Work out the finished part from the listing and answer in its coordinate system (mm). Round coordinates to 2 decimals unless told otherwise and drop trailing zeros. Loops run counter-clockwise (first coordinate to the right, second up) from the corner with the lowest first, then second, coordinate; pieces in that order, holes last. Notation, with made-up numbers: (-5.75, 83) -> (41.25, 83) arc R11 ccw to (41.25, 87) -> close; hole circle Ø7 at (57.5, 10). An arc over 180 degrees is marked (long way). Write item = value, one per line. Start each with the question number.
```python
from build123d import *

# Parameters (mm, degrees)
EXTRUDE_1_DEPTH       = 240
SHEET_START           = -240
SHEET_METAL_1_DEPTH   = 480
SHEET_METAL_1_2_DEPTH = 480
CUT_EXTRUDE_1_REACH   = 247.072
SKETCH_7_R            = 2.5


# Read off the part's stored shape, not the designer's step: Преобразовать-Твердое тело1
with BuildPart() as part:
    # Sketch 1 → Вытянуть-Тонкостенный1 (new, symmetric)
    with BuildSketch(Plane(origin=(0, 0, 0), x_dir=(0, 0, -1), z_dir=(1, 0, 0))):
        Polygon((-19.047619048, 27.896825397), (-19.047619048, 37.896825397), (12.952380952, 37.896825397), (12.952380952, -12.103174603), (2.952380952, -12.103174603), (2.952380952, -10.103174603), (10.952380952, -10.103174603), (10.952380952, 35.896825397), (-17.047619048, 35.896825397), (-17.047619048, 27.896825397), align=None)
    extrude(amount=EXTRUDE_1_DEPTH, both=True)

    # Sheet Metal 1 outline → Sheet Metal 1 (cut)
    with BuildSketch(Plane.YZ.offset(SHEET_START)):
        with BuildLine():
            Line((-12.103174603, -12.952380952), (-8.103174603, -12.952380952))
            ThreePointArc((-8.103174603, -12.952380952), (-10.931601728, -11.780808077), (-12.103174603, -8.952380952))
            Line((-12.103174603, -8.952380952), (-12.103174603, -12.952380952))
        make_face()
        with BuildLine():
            ThreePointArc((33.896825397, 19.047619048), (36.725252521, 17.876046172), (37.896825397, 15.047619048))
            Line((37.896825397, 15.047619048), (37.896825397, 19.047619048))
            Line((37.896825397, 19.047619048), (33.896825397, 19.047619048))
        make_face()
        with BuildLine():
            ThreePointArc((37.896825397, -8.952380952), (36.725252522, -11.780808077), (33.896825397, -12.952380952))
            Line((33.896825397, -12.952380952), (37.896825397, -12.952380952))
            Line((37.896825397, -12.952380952), (37.896825397, -8.952380952))
        make_face()
    extrude(amount=SHEET_METAL_1_DEPTH, mode=Mode.SUBTRACT)

    # Sheet Metal 1 2 outline → Sheet Metal 1 2 (add)
    with BuildSketch(Plane.YZ.offset(SHEET_START)):
        with BuildLine():
            Line((-10.103174603, -10.952380952), (-8.103174603, -10.952380952))
            ThreePointArc((-8.103174603, -10.952380952), (-9.517388166, -10.366594515), (-10.103174603, -8.952380952))
            Line((-10.103174603, -8.952380952), (-10.103174603, -10.952380952))
        make_face()
        with BuildLine():
            ThreePointArc((33.896825397, 17.047619048), (35.311038959, 16.46183261), (35.896825397, 15.047619048))
            Line((35.896825397, 15.047619048), (35.896825397, 17.047619048))
            Line((35.896825397, 17.047619048), (33.896825397, 17.047619048))
        make_face()
        with BuildLine():
            ThreePointArc((35.896825397, -8.952380952), (35.31103896, -10.366594515), (33.896825397, -10.952380952))
            Line((33.896825397, -10.952380952), (35.896825397, -10.952380952))
            Line((35.896825397, -10.952380952), (35.896825397, -8.952380952))
        make_face()
    extrude(amount=SHEET_METAL_1_2_DEPTH)

    # Эскиз7 → Вырез-Вытянуть1 (cut, up to next)
    with BuildSketch(Plane(origin=(0, 0, -12.952380952), x_dir=(-1, 0, 0), z_dir=(0, 0, -1)), mode=Mode.PRIVATE) as cut_extrude_1_sk1:
        with Locations(Location((-207.5, 25.396825397, 0), (0, 0, 90))):
            Circle(SKETCH_7_R)
    cut_extrude_1_tool1 = extrude(cut_extrude_1_sk1.sketch, amount=-CUT_EXTRUDE_1_REACH, mode=Mode.PRIVATE) & part.part
    # Эскиз7 → Вырез-Вытянуть1 (cut, up to next)
    with BuildSketch(Plane(origin=(0, 0, -12.952380952), x_dir=(-1, 0, 0), z_dir=(0, 0, -1)), mode=Mode.PRIVATE) as cut_extrude_1_sk2:
        with Locations(Location((-232.5, 25.396825397, 0), (0, 0, 90))):
            Circle(SKETCH_7_R)
    cut_extrude_1_tool2 = extrude(cut_extrude_1_sk2.sketch, amount=-CUT_EXTRUDE_1_REACH, mode=Mode.PRIVATE) & part.part
    # Эскиз7 → Вырез-Вытянуть1 (cut, up to next)
    with BuildSketch(Plane(origin=(0, 0, -12.952380952), x_dir=(-1, 0, 0), z_dir=(0, 0, -1)), mode=Mode.PRIVATE) as cut_extrude_1_sk3:
        with Locations(Location((-232.5, 0.396825397, 0), (0, 0, 90))):
            Circle(SKETCH_7_R)
    cut_extrude_1_tool3 = extrude(cut_extrude_1_sk3.sketch, amount=-CUT_EXTRUDE_1_REACH, mode=Mode.PRIVATE) & part.part
    # Эскиз7 → Вырез-Вытянуть1 (cut, up to next)
    with BuildSketch(Plane(origin=(0, 0, -12.952380952), x_dir=(-1, 0, 0), z_dir=(0, 0, -1)), mode=Mode.PRIVATE) as cut_extrude_1_sk4:
        with Locations(Location((-207.5, 0.396825397, 0), (0, 0, 90))):
            Circle(SKETCH_7_R)
    cut_extrude_1_tool4 = extrude(cut_extrude_1_sk4.sketch, amount=-CUT_EXTRUDE_1_REACH, mode=Mode.PRIVATE) & part.part
    # Эскиз7 → Вырез-Вытянуть1 (cut, up to next)
    with BuildSketch(Plane(origin=(0, 0, -12.952380952), x_dir=(-1, 0, 0), z_dir=(0, 0, -1)), mode=Mode.PRIVATE) as cut_extrude_1_sk5:
        with Locations(Location((232.5, 25.396825397, 0), (0, 0, 90))):
            Circle(SKETCH_7_R)
    cut_extrude_1_tool5 = extrude(cut_extrude_1_sk5.sketch, amount=-CUT_EXTRUDE_1_REACH, mode=Mode.PRIVATE) & part.part
    # Эскиз7 → Вырез-Вытянуть1 (cut, up to next)
    with BuildSketch(Plane(origin=(0, 0, -12.952380952), x_dir=(-1, 0, 0), z_dir=(0, 0, -1)), mode=Mode.PRIVATE) as cut_extrude_1_sk6:
        with Locations(Location((207.5, 25.396825397, 0), (0, 0, 90))):
            Circle(SKETCH_7_R)
    cut_extrude_1_tool6 = extrude(cut_extrude_1_sk6.sketch, amount=-CUT_EXTRUDE_1_REACH, mode=Mode.PRIVATE) & part.part
    # Эскиз7 → Вырез-Вытянуть1 (cut, up to next)
    with BuildSketch(Plane(origin=(0, 0, -12.952380952), x_dir=(-1, 0, 0), z_dir=(0, 0, -1)), mode=Mode.PRIVATE) as cut_extrude_1_sk7:
        with Locations(Location((207.5, 0.396825397, 0), (0, 0, 90))):
            Circle(SKETCH_7_R)
    cut_extrude_1_tool7 = extrude(cut_extrude_1_sk7.sketch, amount=-CUT_EXTRUDE_1_REACH, mode=Mode.PRIVATE) & part.part
    # Эскиз7 → Вырез-Вытянуть1 (cut, up to next)
    with BuildSketch(Plane(origin=(0, 0, -12.952380952), x_dir=(-1, 0, 0), z_dir=(0, 0, -1)), mode=Mode.PRIVATE) as cut_extrude_1_sk8:
        with Locations(Location((232.5, 0.396825397, 0), (0, 0, 90))):
            Circle(SKETCH_7_R)
    cut_extrude_1_tool8 = extrude(cut_extrude_1_sk8.sketch, amount=-CUT_EXTRUDE_1_REACH, mode=Mode.PRIVATE) & part.part
    add(cut_extrude_1_tool1.solids().sort_by_distance((207.5, 25.396825, -12.952381))[0], mode=Mode.SUBTRACT)
    add(cut_extrude_1_tool2.solids().sort_by_distance((232.5, 25.396825, -12.952381))[0], mode=Mode.SUBTRACT)
    add(cut_extrude_1_tool3.solids().sort_by_distance((232.5, 0.396825, -12.952381))[0], mode=Mode.SUBTRACT)
    add(cut_extrude_1_tool4.solids().sort_by_distance((207.5, 0.396825, -12.952381))[0], mode=Mode.SUBTRACT)
    add(cut_extrude_1_tool5.solids().sort_by_distance((-232.5, 25.396825, -12.952381))[0], mode=Mode.SUBTRACT)
    add(cut_extrude_1_tool6.solids().sort_by_distance((-207.5, 25.396825, -12.952381))[0], mode=Mode.SUBTRACT)
    add(cut_extrude_1_tool7.solids().sort_by_distance((-207.5, 0.396825, -12.952381))[0], mode=Mode.SUBTRACT)
    add(cut_extrude_1_tool8.solids().sort_by_distance((-232.5, 0.396825, -12.952381))[0], mode=Mode.SUBTRACT)


solid = part.part
```
Item 1: Section B-B (z = 7) is taken. Determine the outline of the cut face in (x, y).
Item 2: Find the intervals of material crossed by line 1 along Y through (x, z) = (-232.5, -12.3); line 2 along Y through (x, z) = (207.5, -11.5); line 3 along Z through (x, y) = (-43.5, 30), in increasing order. Write a range as [from, to].
Item 3: Section A-A (x = -59.5) is taken. Determine the outline of the cut face in (y, z), then the cut area to 3 significant figures.
Item 4: Flat-ended cylindrical pins translate along their axes: pin 1 (6 mm diameter, centred on x = -70.5, z = 9, fed in from -Y); pin 2 (5 mm diameter, centred on x = -107, y = 0.5, fed in from +Z); pin 3 (0.6 mm diameter, centred on x = -85, z = 18, fed in from -Y). Find the tip coordinate at first contact, or state that the pin passes through.
Item 5: The mould has two halves that part along Y. Classify faces 1 (the flat face through (3, 35.897, 3)), 2 (the flat face through (3, 37.897, 3)), 3 (the flat face through (240, 20, -12)): pulls with the +Y half, pulls with the -Y half, needs draft (parallel to the pull), parting line crosses it, or undercut.
Worked answers:
q1.outline = (-240, 35.9) -> (240, 35.9) -> (240, 37.9) -> (-240, 37.9) -> close
q2.line_1 = [-10.29, -2.1], [2.9, 22.9], [27.9, 36.09]
q2.line_2 = [-11.19, -2.1], [2.9, 22.9], [27.9, 36.98]
q2.line_3 = [-12.95, -10.95], [17.05, 19.05]
q3.outline = (-12.1, -8.95) arc R4 ccw to (-8.1, -12.95) -> (33.9, -12.95) arc R4 ccw to (37.9, -8.95) -> (37.9, 15.05) arc R4 ccw to (33.9, 19.05) -> (27.9, 19.05) -> (27.9, 17.05) -> (33.9, 17.05) arc R2 cw to (35.9, 15.05) -> (35.9, -8.95) arc R2 cw to (33.9, -10.95) -> (-8.1, -10.95) arc R2 cw to (-10.1, -8.95) -> (-10.1, -2.95) -> (-12.1, -2.95) -> close
q3.area = 184 mm2
q4.pin_1 = 35.9
q4.pin_2 = -10.95
q4.pin_3 = 27.9
q5.face_1 = undercut
q5.face_2 = pulls with the +Y half
q5.face_3 = needs draft
